Check sheet for the modelled part. Datum: model origin and axes. Units: mm. Coordinates: 2 decimals unless noted, no trailing zeros. Loops run counter-clockwise (first coordinate to the right, second up) from the corner with the lowest first, then second, coordinate; pieces in that order, holes last. Notation, with made-up numbers: M -31.5,-23 L -23.5,-23 A15 ccw -23.5,-1 Z; hole C -30,72 d2. An arc over 180 degrees is marked long. Write each question's results on one line, items separated by ' | '. Start each with the question number.
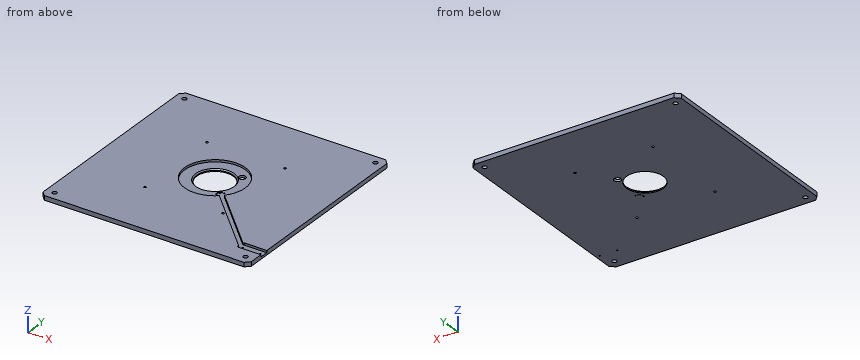
Autodesk Inventor part; units mm, degrees
ref_plane "YZ Plane" through (0, 0, 0) normal (1, 0, 0) x (0, 1, 0)
ref_plane "XZ Plane" through (0, 0, 0) normal (0, 1, 0) x (-1, 0, 0)
ref_plane "XY Plane" through (0, 0, 0) normal (0, 0, 1) x (1, 0, 0)
sketch "Sketch1" plane through (0, 0, 0) normal (0, 0, 1) x (1, 0, 0)
  line L0 (-152.4, 152.4) -> (152.4, 152.4)
  line L1 (152.4, 152.4) -> (152.4, -152.4)
  line L2 (152.4, -152.4) -> (-152.4, -152.4)
  line L3 (-152.4, -152.4) -> (-152.4, 152.4)
  circle A0 centre (0, 0) radius 26.67
  circle A1 centre (-139.7, 139.7) radius 3.2639
  circle A2 centre (139.7, 139.7) radius 3.2639
  circle A3 centre (139.7, -139.7) radius 3.2639
  circle A4 centre (-139.7, -139.7) radius 3.2639
  point P0 (0, 152.4)
  point P1 (-152.4, 0)
  dimension "d0" = 53.34
  dimension "d1" = 304.8
  dimension "d2" = 304.8
  dimension "d3" = 6.5278
  dimension "d4" = 6.5278
  dimension "d5" = 6.5278
  dimension "d6" = 6.5278
  dimension "d7" = 279.4
  dimension "d8" = 139.7
  dimension "d9" = 279.4
  dimension "d10" = 139.7
extrude "Extrusion1" add sketch "Sketch1" along normal blind 6.35
chamfer "Chamfer1" distance 6.35 angle 45 4 edges at (152.4, 152.4, 3.175) (152.4, -152.4, 3.175) (-152.4, 152.4, 3.175) (-152.4, -152.4, 3.175)
sketch "Sketch10" plane through (0, 0, 6.35) normal (0, 0, 1) x (1, 0, 0)
  line L0 (-213.36, 0) -> (213.36, 0) construction
  line L1 (0, -213.36) -> (0, 213.36) construction
  line L2 (-81.3558, 81.3558) -> (81.3558, -81.3558) construction
  line L3 (15.2664, -26.0427) -> (26.0427, -15.2664) construction
  line L4 (26.0427, -15.2664) -> (33.2269, -22.4506) construction
  line L5 (27.8388, -27.8388) -> (22.4506, -33.2269) construction
  line L6 (22.4506, -33.2269) -> (15.2664, -26.0427) construction
  circle A0 centre (0, 0) radius 26.67
  line L7 (18.8585, -29.6348) -> (29.6348, -18.8585) construction
  line L8 (152.4, 146.05) -> (152.4, -146.05)
  line L9 (152.4, -112.6871) -> (120.0658, -112.6871)
  line L10 (116.8908, -115.8621) -> (116.8908, -122.2375)
  line L11 (120.0658, -125.4125) -> (152.4, -125.4125)
  line L12 (152.4, -125.4125) -> (152.4, -112.6871)
  arc A1 (120.0658, -112.6871) -> (116.8908, -115.8621) centre (120.0658, -115.8621) ccw
  arc A2 (116.8908, -122.2375) -> (120.0658, -125.4125) centre (120.0658, -122.2375) ccw
  line L13 (146.05, -152.4) -> (-146.05, -152.4)
  line L14 (118.491, -123.8123) -> (150.241, -123.8123) construction
  line L15 (150.241, -123.8123) -> (150.241, -114.2873) construction
  line L16 (150.241, -114.2873) -> (118.491, -114.2873) construction
  line L17 (118.491, -114.2873) -> (118.491, -123.8123) construction
  line L18 (134.366, -114.2873) -> (134.366, -123.8123) construction
  line L19 (118.491, -119.0498) -> (150.241, -119.0498) construction
  arc A3 (33.5957, -29.1055) -> (29.1055, -33.5957) centre (0, 0) ccw
  line L20 (29.1055, -33.5957) -> (116.8908, -121.3809)
  line L21 (33.5957, -29.1055) -> (117.9685, -113.4784)
  line L22 (21.9118, -20.8342) -> (24.0671, -22.9895)
  line L23 (24.0671, -22.9895) -> (22.9895, -24.0671)
  line L24 (22.9895, -24.0671) -> (20.8342, -21.9118)
  line L25 (20.8342, -21.9118) -> (21.9118, -20.8342)
  line L26 (21.373, -21.373) -> (23.5283, -23.5283) construction
  line L27 (20.1158, -22.6302) -> (22.271, -24.7855)
  line L28 (19.0381, -23.7079) -> (20.1158, -22.6302)
  line L29 (21.1934, -25.8631) -> (19.0381, -23.7079)
  line L30 (22.271, -24.7855) -> (21.1934, -25.8631)
  line L31 (22.6302, -20.1158) -> (23.7079, -19.0381)
  line L32 (24.7855, -22.271) -> (22.6302, -20.1158)
  line L33 (23.7079, -19.0381) -> (25.8631, -21.1934)
  line L34 (25.8631, -21.1934) -> (24.7855, -22.271)
  point P0 (22.3249, -22.3249)
  point P1 (20.6546, -27.8388)
  point P2 (27.8388, -20.6546)
  point P3 (121.666, -119.0498)
  point P4 (147.066, -119.0498)
  point P5 (20.5289, -24.121)
  point P6 (24.121, -20.5289)
  point P7 (19.577, -23.1691)
  point P8 (21.7322, -25.3243)
  point P9 (23.1691, -19.577)
  point P10 (25.3243, -21.7322)
  dimension "d84" = 45
  dimension "d85" = 10.16
  dimension "d86" = 15.24
  dimension "d87" = 39.37
  dimension "d90" = 2.3622
  dimension "d91" = 10.16
  dimension "d101" = 3.175
  dimension "d120" = 31.75
  dimension "d121" = 9.525
  dimension "d122" = 25.4
  dimension "d124" = 33.3502
  dimension "d125" = 1.6002
  dimension "d126" = 1.6002
  dimension "d128" = 2.159
  dimension "d156" = 88.9
  dimension "d159" = 6.35
  dimension "d163" = 2.3622
  dimension "d164" = 2.3622
  dimension "d165" = 2.54
  dimension "d166" = 2.54
  dimension "d167" = 3.048
  dimension "d168" = 1.524
  dimension "d172" = 2.54
  dimension "d179" = 2.54
  dimension "d185" = 1.016
hole "Hole8" at (22.3249, -22.3249, 6.35) at (20.5289, -24.121, 6.35) at (24.121, -20.5289, 6.35) direction (0, 0, -1) diameter 1.27 end through all
hole "Hole9" at (20.6546, -27.8388, 6.35) at (27.8388, -20.6546, 6.35) at (121.666, -119.0498, 6.35) at (147.066, -119.0498, 6.35) direction (0, 0, -1) diameter 1.7018 end through all
extrude "Extrusion5" cut sketch "Sketch10" against normal blind 3.175 contours A0 | L8 L11 A2 L10 A1 L9 | A1 L10 L20 A3 L21 | L22 L23 L24 L25 | L27 L30 L29 L28 | L31 L33 L34 L32
sketch "Sketch11" plane through (0, 0, 6.35) normal (0, 0, 1) x (1, 0, 0)
  line L0 (-213.36, 0) -> (213.36, 0) construction
  line L1 (0, -213.36) -> (0, 213.36) construction
  line L2 (-84.555, -84.555) -> (84.555, 84.555) construction
  circle A0 centre (22.4506, 22.4506) radius 1.9812 construction
  circle A1 centre (26.0427, 26.0427) radius 0.8509 construction
  circle A2 centre (23.8516, 23.8516) radius 4.9022
  point P0 (0, 0)
  dimension "d130" = 45
  dimension "d135" = 3.9624
  dimension "d136" = 1.7018
  dimension "d142" = 31.75
  dimension "d143" = 5.08
  dimension "d157" = 9.8044
  dimension "d158" = 33.7312
extrude "Extrusion6" cut sketch "Sketch11" against normal through all
sketch "Sketch12" plane through (0, 0, 0) normal (0, 0, -1) x (-1, 0, 0)
  line L0 (-57.15, 66.675) -> (57.15, 66.675) construction
  line L1 (57.15, 66.675) -> (57.15, -66.675) construction
  line L2 (57.15, -66.675) -> (-57.15, -66.675) construction
  line L3 (-57.15, -66.675) -> (-57.15, 66.675) construction
  line L4 (-57.15, 66.675) -> (57.15, -66.675) construction
  point P0 (0, 0)
  point P1 (0, 0)
  dimension "d147" = 133.35
  dimension "d148" = 114.3
hole "Hole10" at (-57.15, 66.675, 0) at (-57.15, -66.675, 0) at (57.15, -66.675, 0) at (57.15, 66.675, 0) direction (0, 0, 1) diameter 3.302 end through all
chamfer "Chamfer2" distance 1.6002 angle 45 1 edges at (-26.67, 0, 3.175)
extrude "Extrusion7" cut sketch "Sketch10" against normal blind 4.191 contours L22 L23 L24 L25 | L27 L30 L29 L28 | L31 L33 L34 L32
equation "\"d4\" = d3"
equation "\"d5\" = d3"
equation "\"d6\" = d3"
equation "\"d126\" = d125"
properties part number "J002949" material "ALUMINUM, 6061-T651"
Item 1: Thickness scan on line 1 (X direction, y = 137, z = 2.5); line 2 (Y direction, x = 133.5, z = 5); line 3 (X direction, y = -3.5, z = 2.25). Record the ranges inside material, lowest first.
Item 2: Depth check by flat-ended pin: P1, Ø3.5, axis at x = 24.5, y = -20.5, coming from the +Z side (3 decimals); P2, Ø1.4, axis at x = 20.65, y = -27.84, coming from the +Z side; P3, Ø0.7, axis at y = -122, z = 4.5, coming from the +X side; P4, Ø5.5, axis at x = 57.15, y = 66.675, coming from the +Z side. Enter the tip coordinate at first touch or a pass-through.
Item 3: Section check A-A (x = 0). Record the cut outline in (y, z) (3 decimals).
Item 4: Section check C-C (z = 4.25). State how many separate pieces and enclosed holes the cut face has, plus the area to 3 significant figures.
Computed values:
1) line 1: x = -152.4 to -141.53, -137.87 to 137.87, 141.53 to 152.4 | line 2: y = -152.4 to -125.41, -112.69 to 152.4 | line 3: x = -152.4 to -27.12, 27.12 to 152.4
2) P1: stops at z = 3.175 | P2: passes through | P3: stops at x = 116.89 | P4: stops at z = 6.35
3) outline: M -152.4,0 L -26.67,0 L -26.67,1.575 L -28.27,3.175 L -44.45,3.175 L -44.45,6.35 L -152.4,6.35 Z; M 26.67,0 L 152.4,0 L 152.4,6.35 L 44.45,6.35 L 44.45,3.175 L 28.27,3.175 L 26.67,1.575 Z
4) separate pieces: 1 | enclosed holes: 8 | area: 85,200 mm²
